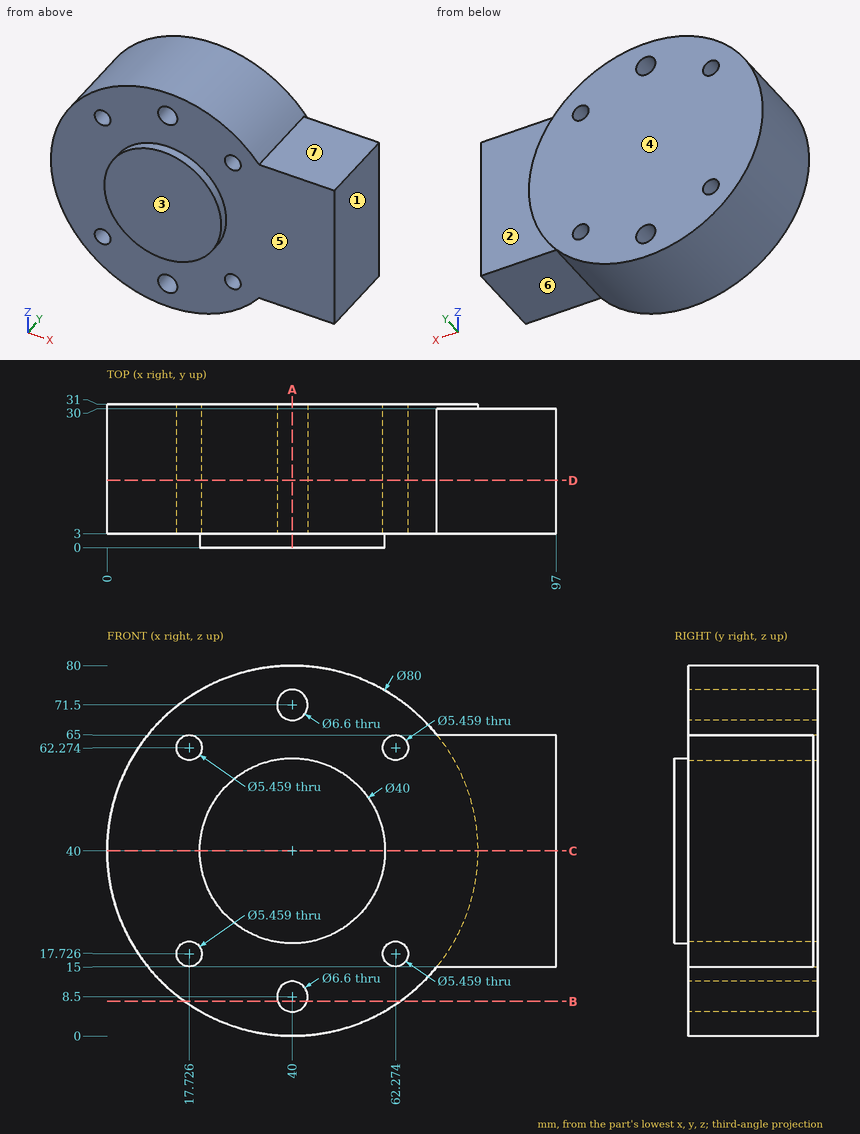
Geometry check sheet. Reference: drawing and pictorial views, mm from the part's lowest x, y, z. A direction names the side the tool comes from. Coordinates: 2 decimals unless noted, no trailing zeros. Order: outer loops, then holes, each group sorted by start corner. A loop starts at its lowest first (then second) coordinate and runs counter-clockwise, first axis right, second up.
Item 1: Depth check by flat-ended pin: pin 1 (10 mm diameter, centred on x = 28, y = 7, fed in from -Z); pin 2 (6.5 mm diameter, centred on x = 62.27, z = 62.27, fed in from -Y); pin 3 (12 mm diameter, centred on y = 22.5, z = 13, fed in from -X). Enter the tip coordinate at first touch or a pass-through.
Item 2: Section check D-D (y = 14.5). Enter the section's corners in (x, z) (1 decimal), plus the area to 3 significant figures.
Item 3: Section check A-A (x = 40). Enter the section's corners in (y, z), plus the area to 3 significant figures.
Item 4: Section check C-C (z = 40). Enter the section's corners in (x, y).
Item 5: Scan lines: line 1 along Z through (x, y) = (40, 9.5); line 2 along X through (y, z) = (11, 62); line 3 along Z through (x, y) = (16, 27). Record each from-to range of solid material in increasing order.
Item 6: Section check B-B (z = 7.5). Enter the section's corners in (x, y) (1 decimal).
Item 7: Tool access check on the marked faces 4, 5, 6 and 7. Record the directions out of +Z, -Z, +X, -X, +Y, -Y that give a thin tool (end or side, any length) a straight path to the whole face; none if there is none.
Item 8: Mould release check, pull along Y, two halves, no side actions. Record for the marked faces 1, 2 and 3: released by +Y, released by -Y, zero draft, split by the parting line, or undercut.
Check sheet entries:
1. pin 1: stops at z = 0.62
1. pin 2: stops at y = 3
1. pin 3: stops at x = 5.96
2. outline: (71.2, 15) - (97, 15) - (97, 65) - (71.2, 65) arc R40 ccw (long way) to start; hole circle Ø5.5 at (17.7, 17.7); hole circle Ø5.5 at (17.7, 62.3); hole circle Ø6.6 at (40, 8.5); hole circle Ø6.6 at (40, 71.5); hole circle Ø5.5 at (62.3, 17.7); hole circle Ø5.5 at (62.3, 62.3)
2. area: 5,850 mm2
3. outline: (0, 20) - (3, 20) - (3, 11.8) - (31, 11.8) - (31, 68.2) - (3, 68.2) - (3, 60) - (0, 60) - close; (3, 0) - (31, 0) - (31, 5.2) - (3, 5.2) - close; (3, 74.8) - (31, 74.8) - (31, 80) - (3, 80) - close
3. area: 1,990 mm2
4. outline: (0, 3) - (20, 3) - (20, 0) - (60, 0) - (60, 3) - (97, 3) - (97, 30) - (80, 30) - (80, 31) - (0, 31) - close
5. line 1: z = 0 to 5.2, 11.8 to 68.2, 74.8 to 80
5. line 2: x = 6.59 to 15.01, 20.44 to 59.56, 64.99 to 97
5. line 3: z = 8 to 15.61, 19.84 to 60.16, 64.39 to 72
6. outline: (16.7, 3) - (36.9, 3) - (36.9, 31) - (16.7, 31) - close; (43.1, 3) - (63.3, 3) - (63.3, 31) - (43.1, 31) - close
7. face 4: +Z, -Z, +X, -X, +Y
7. face 5: -Y
7. face 6: -Z, +X, +Y, -Y
7. face 7: +Z, +X, +Y, -Y
8. face 1: zero draft
8. face 2: released by +Y
8. face 3: released by -Y
